from build123d import *

# Parameters (mm, degrees)
F0_W           = 100
F0_H           = 100
F0_R           = 22.5
F1_DEPTH       = 10
F0_R_2         = 11.15
F0_R_3         = 4.75
F2_DEPTH       = 5
F0_R_4         = 14.3
F3_DEPTH       = 22
F4_DEPTH       = 28
F6_D           = 5
F6_CBORE_D     = 9
F6_CBORE_DEPTH = 1.5
F7_R           = 3
F8_W           = 4
F8_H           = 30
F9_DEPTH       = 5
F5_R           = 2.5
F10_DEPTH      = 10.001


with BuildPart() as f1:
    # F0 (on Top) → F1 (new body)
    with BuildSketch(Plane.XY):
        Rectangle(F0_W, F0_H)
        Circle(F0_R, mode=Mode.SUBTRACT)
    extrude(amount=F1_DEPTH)



with BuildPart() as f2:
    # F0 (on Top) → F2 (new body)
    with BuildSketch(Plane.XY):
        Circle(F0_R_2)
        Circle(F0_R_3, mode=Mode.SUBTRACT)
    extrude(amount=F2_DEPTH)

    # F0 (on Top) → F3 (join)
    with BuildSketch(Plane.XY):
        Circle(F0_R_4)
        Circle(F0_R_2, mode=Mode.SUBTRACT)
    extrude(amount=F3_DEPTH)


with BuildPart() as f1_1:
    add(f1.part)

    add(f2.part)  # F4 merges F2
    # F0 (on Top) → F4 (join)
    with BuildSketch(Plane.XY):
        Circle(F0_R)
        Circle(F0_R_4, mode=Mode.SUBTRACT)
    extrude(amount=F4_DEPTH)

    # F6 (through all)
    with Locations(Plane.XY.offset(10)):
        with Locations((-40, 40), (40, 40), (40, -40), (-40, -40)):
            CounterBoreHole(F6_D / 2, F6_CBORE_D / 2, F6_CBORE_DEPTH)

    # F7
    f7_edges = [f1_1.edges().sort_by_distance(p)[0] for p in [
        (-50, 0, 10),
        (0, 50, 10),
        (50, 0, 10),
        (0, -50, 10),
        (-22.5, 0, 10),
        (-22.5, 0, 28),
    ]]
    fillet(f7_edges, radius=F7_R)

    # F8 (on face) → F9 (cut)
    with BuildSketch(Plane.XY.offset(28)):
        with Locations((0, -15)):
            Rectangle(F8_W, F8_H)
    extrude(amount=-F9_DEPTH, mode=Mode.SUBTRACT)

    # F5 (on face) → F10 (cut, through all)
    with BuildSketch(Plane.XY.offset(10)):
        with Locations((0, -35)):
            Circle(F5_R)
    extrude(amount=-F10_DEPTH, mode=Mode.SUBTRACT)


solid = f1_1.part
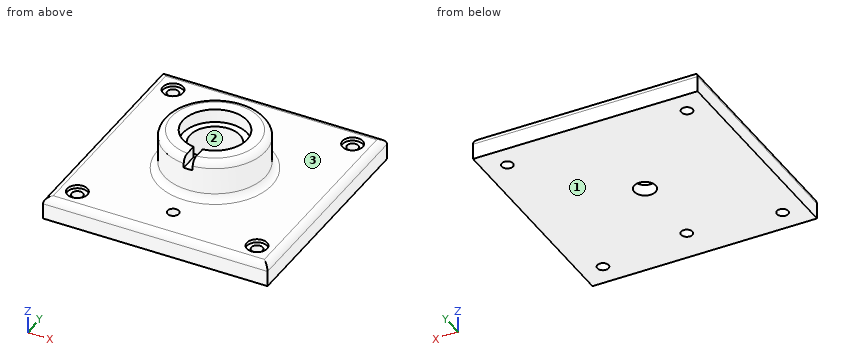
The listing builds one solid part. Answer for the finished solid, in the listing's coordinates (mm). Face numbers are marked on the shaded views. Coordinates: 2 decimals unless noted, no trailing zeros. Order: outer loops, then holes, each group sorted by start corner. A loop starts at its lowest first (then second) coordinate and runs counter-clockwise, first axis right, second up. Notation, with made-up numbers: (1, 81) -> (8, 81) arc R22 cw to (8, 99) -> close; hole circle Ø5 at (69.5, 21). An arc over 180 degrees is marked (long way). Answer in a Markdown table with one row per item. Add a question column.
Item 1: Find section C-C (y = 40). Write down the section's boundary in (x, z).
Item 2: Determine the mould class of the marked faces 1, 2 and 3 for opening direction Z: +Z half, -Z half, draft (parallel to the pull), parting line (faces both ways), or undercut.
Item 3: Find section A-A (x = 0). State how many separate pieces and enclosed holes the cut face has, then the cut area to 3 significant figures.
Item 4: Find the intervals of material crossed by L1, parallel to Y at x = 0, z = 5.5; L2, parallel to Y at x = -40, z = 6.5; L3, parallel to Z at x = -15, y = 44, in increasing order. Write a range as from..to.
Item 5: Find section B-B (y = 0). Write down the section's boundary in (x, z), then the cut area to 3 significant figures.
Item 6: Find section D-D (z = 16.25). Write down the section's boundary in (x, y), then the cut area to 3 significant figures.
Item 7: Each of these flat-tipped pins is pushed along its axis until it touches: P1, Ø3, axis at x = 40, y = 40, coming from the +Z side; P2, Ø17, axis at x = 0, y = 0, coming from the +Z side; P3, Ø4, axis at x = -2.5, z = 14, coming from the +Y side; P4, Ø6.5, axis at x = 40, y = -40, coming from the +Z side. Where does it stop, or does it pass through?
Result set:
| question | item | result |
|---|---|---|
| 1 | outline | (-50, 0) -> (-42.5, 0) -> (-42.5, 8.5) -> (-44.5, 8.5) -> (-44.5, 10) -> (-47, 10) arc R3 ccw to (-50, 7) -> close; (-37.5, 0) -> (37.5, 0) -> (37.5, 8.5) -> (35.5, 8.5) -> (35.5, 10) -> (-35.5, 10) -> (-35.5, 8.5) -> (-37.5, 8.5) -> close; (42.5, 0) -> (50, 0) -> (50, 7) arc R3 ccw to (47, 10) -> (44.5, 10) -> (44.5, 8.5) -> (42.5, 8.5) -> close |
| 2 | face 1 | -Z half |
| 2 | face 2 | draft |
| 2 | face 3 | +Z half |
| 3 | separate pieces | 3 |
| 3 | enclosed holes | 0 |
| 3 | area | 1,120 mm² |
| 4 | L1 | y = -50..-37.5, -32.5..-11.15, 11.15..50 |
| 4 | L2 | y = -50..-42.5, -37.5..37.5, 42.5..50 |
| 4 | L3 | z = 0..10 |
| 5 | outline | (-50, 0) -> (-4.75, 0) -> (-4.75, 5) -> (-11.15, 5) -> (-11.15, 22) -> (-14.3, 22) -> (-14.3, 28) -> (-19.5, 28) arc R3 ccw to (-22.5, 25) -> (-22.5, 13) arc R3 cw to (-25.5, 10) -> (-47, 10) arc R3 ccw to (-50, 7) -> close; (4.75, 0) -> (50, 0) -> (50, 7) arc R3 ccw to (47, 10) -> (25.5, 10) arc R3 cw to (22.5, 13) -> (22.5, 25) arc R3 ccw to (19.5, 28) -> (14.3, 28) -> (14.3, 22) -> (11.15, 22) -> (11.15, 5) -> (4.75, 5) -> close |
| 5 | area | 1,210 mm² |
| 6 | outline | circle Ø45 at (0, 0); hole circle Ø22.3 at (0, 0) |
| 6 | area | 1,200 mm² |
| 7 | P1 | passes through |
| 7 | P2 | stops at z = 5 |
| 7 | P3 | stops at y = 22.56 |
| 7 | P4 | stops at z = 8.5 |
